For this review, take the finished solid that the model builds, in its own axes (mm). Face numbers are marked on the shaded views. A direction names the side the tool comes from. Give positions to 0.01 mm unless a question says otherwise; leave off trailing zeros. Order: outer loops, then holes, each group sorted by start corner. A loop starts at its lowest first (then second) coordinate and runs counter-clockwise, first axis right, second up.
Autodesk Inventor part; units mm, degrees
ref_plane "YZ Plane" through (0, 0, 0) normal (1, 0, 0) x (0, 1, 0)
ref_plane "XZ Plane" through (0, 0, 0) normal (0, 1, 0) x (-1, 0, 0)
ref_plane "XY Plane" through (0, 0, 0) normal (0, 0, 1) x (1, 0, 0)
sketch "Sketch1" plane through (0, 0, 0) normal (0, 1, 0) x (-1, 0, 0)
  point P0 (0, 0)
sketch "Sketch2" plane through (0, 0, 0) normal (0, 1, 0) x (-1, 0, 0)
  line L0 (23.25, -20.5) -> (-23.25, -20.5)
  line L1 (-23.25, -20.5) -> (-23.25, 20.5)
  line L2 (-23.25, 20.5) -> (23.25, 20.5)
  line L3 (23.25, 20.5) -> (23.25, -20.5)
  line L4 (23.25, -20.5) -> (-23.25, 20.5) construction
  line L5 (-23.25, -20.5) -> (23.25, 20.5) construction
  point P0 (0, 0)
  dimension "d0" = 46.5
  dimension "d1" = 41
extrude "Extrusion1" add sketch "Sketch2" along normal blind 0.5
sketch "Sketch3" plane through (0, 0.5, 0) normal (0, 1, 0) x (1, 0, 0)
  line L0 (-13, -9) -> (13, -9)
  line L1 (13, -9) -> (13, 9)
  line L2 (13, 9) -> (-13, 9)
  line L3 (-13, 9) -> (-13, -9)
  line L4 (-13, -9) -> (13, 9) construction
  line L5 (13, -9) -> (-13, 9) construction
  point P0 (0, 0)
  dimension "d4" = 26
  dimension "d5" = 18
extrude "Extrusion2" cut sketch "Sketch3" against normal blind 25.4
sketch "Sketch4" plane through (0, 0.5, 0) normal (0, 1, 0) x (1, 0, 0)
  line L0 (-23.25, 20.5) -> (-23.25, -20.5)
  line L1 (23.25, -20.5) -> (23.25, 20.5)
  line L2 (-23.25, -20.5) -> (23.25, -20.5)
  line L3 (23.25, -20.5) -> (23.25, -17.4625)
  line L4 (23.25, -17.4625) -> (-23.25, -17.4625)
  line L5 (-23.25, -17.4625) -> (-23.25, -20.5)
  point P0 (0, 0)
extrude "Extrusion3" add sketch "Sketch4" along normal blind 46.9
sketch "Sketch5" plane through (0, 0.5, 0) normal (0, 1, 0) x (1, 0, 0)
  line L0 (-23.25, 20.5) -> (-23.25, -17.4625)
  line L1 (-23.25, 20.5) -> (23.25, 20.5)
  line L2 (23.25, 20.5) -> (23.25, 17.4625)
  line L3 (23.25, 17.4625) -> (-23.25, 17.4625)
  line L4 (-23.25, 17.4625) -> (-23.25, 20.5)
  point P0 (0, 0)
extrude "Extrusion4" add sketch "Sketch5" along normal blind 46.9
sketch "Sketch6" plane through (23.25, 0.5, 17.4625) normal (0, 0, -1) x (-1, 0, 0)
  point P0 (23.25, -0.5)
sketch "Sketch7" plane through (23.25, 0.5, 17.4625) normal (0, 0, -1) x (-1, 0, 0)
  point P0 (23.25, -0.5)
sketch "Sketch8" plane through (23.25, 0.5, 17.4625) normal (0, 0, -1) x (-1, 0, 0)
  line L0 (46.5, 0) -> (46.5, 46.9)
  line L1 (0, 0) -> (0, 46.9)
  line L2 (46.5, 46.9) -> (0, 46.9)
  line L3 (0, 46.9) -> (0, 43.8105)
  line L4 (0, 43.8105) -> (46.5, 43.8105)
  line L5 (46.5, 43.8105) -> (46.5, 46.9)
  point P0 (23.25, -0.5)
extrude "Extrusion5" add sketch "Sketch8" along normal blind 35
sketch "Sketch9" plane through (0, 47.4, 0) normal (0, 1, 0) x (1, 0, 0)
  line L0 (-13, -9) -> (-13, 9)
  line L1 (13, 9) -> (-13, 9)
  line L2 (-13, 9) -> (-13, -9)
  line L3 (-13, -9) -> (13, -9)
  line L4 (13, -9) -> (13, 9)
  line L5 (13, 9) -> (-13, -9) construction
  line L6 (-13, 9) -> (13, -9) construction
  point P0 (0, 0)
sketch "Sketch10" plane through (0, 0.5, 0) normal (0, 1, 0) x (1, 0, 0)
  point P0 (0, 0)
sketch "Sketch11" plane through (0, 0.5, 0) normal (0, 1, 0) x (1, 0, 0)
  line L0 (-23.25, -17.4625) -> (23.25, -17.4625)
  line L1 (-23.25, -17.4625) -> (-18.283, -17.4625)
  line L2 (-18.283, -17.4625) -> (-18.283, 17.4625)
  line L3 (-18.283, 17.4625) -> (-23.25, 17.4625)
  line L4 (-23.25, 17.4625) -> (-23.25, -17.4625)
  point P0 (0, 0)
extrude "Extrusion6" add sketch "Sketch11" along normal blind 2.9718
extrude "Extrusion7" cut sketch "Sketch9" against normal blind 4.9657
sketch "Sketch12" plane through (0, 0.5, 0) normal (0, 1, 0) x (1, 0, 0)
  point P0 (0, 0)
sketch "Sketch14" plane through (-18.283, 0.5, 17.4625) normal (1, 0, 0) x (0, 0, -1)
  line L0 (0, 2.9718) -> (0, 43.8105)
  line L1 (34.925, 0) -> (34.925, 43.8105)
  line L2 (0, 2.9718) -> (34.925, 2.9718)
  line L3 (34.925, 2.9718) -> (34.925, 0)
  line L4 (34.925, 0) -> (0, 0)
  line L5 (0, 0) -> (0, 2.9718)
  point P0 (17.4625, -0.5)
extrude "Extrusion9" add sketch "Sketch14" along normal blind 5.08
sketch "Sketch15" plane through (-13.203, 0.5, 17.4625) normal (1, 0, 0) x (0, 0, -1)
  line L0 (0, 0) -> (0, 43.8105)
  line L1 (8.4625, 0) -> (26.4625, 0)
  line L2 (0, 3.1096) -> (8.4625, 3.1096)
  line L3 (8.4625, 3.1096) -> (8.4625, 0)
  line L4 (8.4625, 0) -> (0, 0)
  line L5 (0, 0) -> (0, 3.1096)
  point P0 (17.4625, -0.5)
extrude "Extrusion10" add sketch "Sketch15" along normal blind 36.83
properties part number "ChamberSurface"
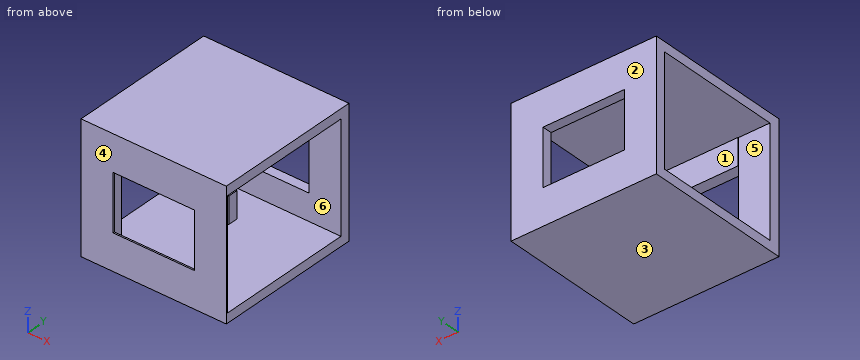
1) Clearance check with flat-ended pins moving along their axes: pin 1 (12 mm diameter, centred on x = -7, z = 8, fed in from -Y); pin 2 (3.5 mm diameter, centred on y = 1.5, z = -3.5, fed in from +X); pin 3 (10.5 mm diameter, centred on x = -6.5, z = -2.5, fed in from -Y). State where each tip first meets the part, or that it passes through.
Answer sheet:
pin 1: stops at y = 0
pin 2: stops at x = 23.25
pin 3: passes through
2) We need section D-D on x = 9. Give the boundary of the cut face in (y, z).
Answer sheet:
outline: (0, -20.5) - (47.4, -20.5) - (47.4, -9) - (44.31, -9) - (44.31, -17.46) - (0.5, -17.46) - (0.5, -9) - (0, -9) - close; (0, 9) - (3.61, 9) - (3.61, 17.46) - (44.31, 17.46) - (44.31, 9) - (47.4, 9) - (47.4, 20.5) - (0, 20.5) - close
3) We need section B-B on x = 14. Give the boundary of the cut face in (y, z).
Answer sheet:
outline: (0, -20.5) - (47.4, -20.5) - (47.4, 20.5) - (0, 20.5) - close; hole (0.5, -17.46) - (44.31, -17.46) - (44.31, 17.46) - (3.61, 17.46) - (3.61, 9) - (0.5, 9) - close
4) We need section C-C on y = 12.5. Give the boundary of the cut face in (x, z), then the cut area to 3 significant figures.
Answer sheet:
outline: (-23.25, -20.5) - (23.25, -20.5) - (23.25, -17.46) - (-23.25, -17.46) - close; (-23.25, 17.46) - (23.25, 17.46) - (23.25, 20.5) - (-23.25, 20.5) - close
area: 282 mm2
5) We need section A-A on z = 10. Give the boundary of the cut face in (x, y), then the cut area to 3 significant figures.
Answer sheet:
outline: (-23.25, 0) - (23.25, 0) - (23.25, 0.5) - (23.63, 0.5) - (23.63, 3.61) - (-13.2, 3.61) - (-13.2, 3.47) - (-23.25, 3.47) - close; (-23.25, 44.31) - (23.25, 44.31) - (23.25, 47.4) - (-23.25, 47.4) - close
area: 311 mm2
6) To check wall thickness, follow line 1 (Z direction, x = 12.5, y = 37); line 2 (Y direction, x = -16, z = -15); line 3 (Y direction, x = -1.5, z = 9.5). State the ranges of each line that lie inside material, in increasing order.
Answer sheet:
line 1: z = -20.5 to -17.46, 17.46 to 20.5
line 2: y = 0 to 3.47, 44.31 to 47.4
line 3: y = 0 to 3.61, 44.31 to 47.4
7) Draft analysis for pull direction Y (two halves, no side actions). For the marked faces 1, 2 and 3, state which applies: +Y half, -Y half, draft (parallel to the pull), parting line (faces both ways), or undercut.
Answer sheet:
face 1: undercut
face 2: +Y half
face 3: draft
8) Tool access review of the marked faces 4, 5 and 6: name each direction out of +Z, -Z, +X, -X, +Y, -Y from which nothing blocks a thin tool from reaching the whole face with its end or side.
Answer sheet:
face 4: +Z, -Z, +X, -X, -Y
face 5: -X
face 6: +X, -X
